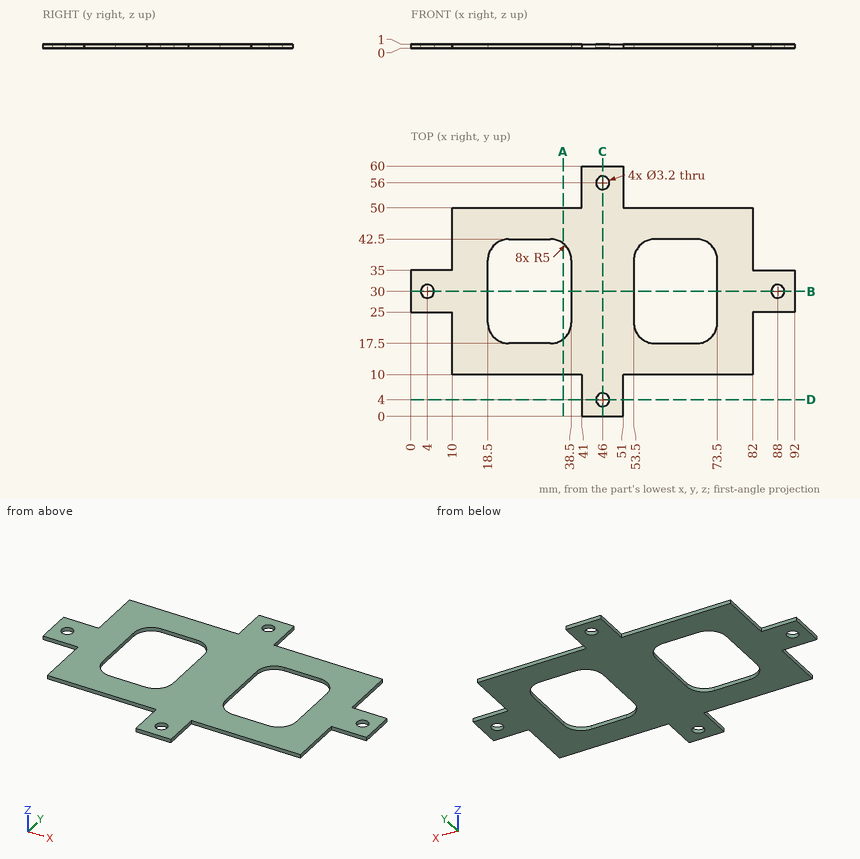
Job drawing, mm, ordinate dimensions from the low corner. One solid piece. Coordinates: 2 decimals unless noted, no trailing zeros. Order: outer loops, then holes, each group sorted by start corner. A loop starts at its lowest first (then second) coordinate and runs counter-clockwise, first axis right, second up. Notation, with made-up numbers: M 49,29 L 77,29 A29 cw 77,49 Z; hole C 0.25,-16 d6. An arc over 180 degrees is marked long. One line per question, with ' | ' between items.
Q1. Slice it at C-C (x = 46). Give the cut face in (y, z), and give its area (3 significant figures).
A:
outline: M 0,0 L 2.4,0 L 2.4,1 L 0,1 Z; M 5.6,0 L 54.4,0 L 54.4,1 L 5.6,1 Z; M 57.6,0 L 60,0 L 60,1 L 57.6,1 Z | area: 53.6 mm^2
Q2. Pin check, flat tips, straight feed: P1, Ø0.5, axis at x = 26.5, z = 0.5, coming from the +Y side; P2, Ø2.5, axis at x = 46, y = 4, coming from the +Z side. Stop position of each tip, or through.
A:
P1: stops at y = 50 | P2: passes through
Q3. Drill centre lines: line 1 (X direction, y = 26, z = 0.95); line 2 (Y direction, x = 46, z = 0.45); line 3 (Y direction, x = 4, z = 0.3). Where is each one in solid material? Low to high.
A:
line 1: x = 0 to 18.5, 38.5 to 53.5, 73.5 to 92 | line 2: y = 0 to 2.4, 5.6 to 54.4, 57.6 to 60 | line 3: y = 25 to 28.4, 31.6 to 35
Q4. Slice it at D-D (y = 4). Give the cut face in (x, z).
A:
outline: M 41,0 L 44.4,0 L 44.4,1 L 41,1 Z; M 47.6,0 L 51,0 L 51,1 L 47.6,1 Z
Q5. Slice it at A-A (x = 36.5). Give the cut face in (y, z), and give its area (3 significant figures).
A:
outline: M 10,0 L 18.5,0 L 18.5,1 L 10,1 Z; M 41.5,0 L 50,0 L 50,1 L 41.5,1 Z | area: 17.0 mm^2
Q6. Slice it at B-B (y = 30). Give the cut face in (x, z).
A:
outline: M 0,0 L 2.4,0 L 2.4,1 L 0,1 Z; M 5.6,0 L 18.5,0 L 18.5,1 L 5.6,1 Z; M 38.5,0 L 53.5,0 L 53.5,1 L 38.5,1 Z; M 73.5,0 L 86.4,0 L 86.4,1 L 73.5,1 Z; M 89.6,0 L 92,0 L 92,1 L 89.6,1 Z
